Can you work these out from the model? Positions are in its coordinate system, mm. Give positions to 0.01 mm unless a question says otherwise; leave off trailing zeros. Write each loop counter-clockwise with the first axis right and the second up, starting at its lowest first coordinate (ties: lowest second). Pieces come first, ordered by that corner, then holes. Notation, with made-up numbers: M 50.5,-17.5 L 76.5,-17.5 A23 cw 76.5,7.5 Z; hole C -25,10 d5. An arc over 180 degrees is marked long. Write each question's results on one line, items separated by ' | '.
from build123d import *

# Parameters (mm, degrees)
SKETCH1_R           = 1.75
BOSS_EXTRUDE1_DEPTH = 4
SKETCH2_W           = 130
SKETCH2_H           = 10
BOSS_EXTRUDE2_DEPTH = 0.5
CUT_EXTRUDE1_DEPTH  = 2
SKETCH4_R           = 1.624205192
BOSS_EXTRUDE3_DEPTH = 4


with BuildPart() as part:
    # Sketch1 → Boss-Extrude1 (new body)
    with BuildSketch(Plane(origin=(0, 0, 0), x_dir=(1, 0, 0), z_dir=(0, 1, 0))):
        with BuildLine():
            ThreePointArc((75, 2), (74.121320344, 4.121320344), (72, 5))
            Line((72, 5), (-72, 5))
            ThreePointArc((-72, 5), (-74.121320344, 4.121320344), (-75, 2))
            Line((-75, 2), (-75, -5))
            Line((-75, -5), (75, -5))
            Line((75, -5), (75, 2))
        make_face()
        with Locations(Location((-70, 0, 0), (0, 0, 270))):
            Circle(SKETCH1_R, mode=Mode.SUBTRACT)
        with BuildLine():
            ThreePointArc((61.75, 0), (61.237436867, -1.237436867), (60, -1.75))
            Line((60, -1.75), (-60, -1.75))
            ThreePointArc((-60, -1.75), (-61.75, 0), (-60, 1.75))
            Line((-60, 1.75), (60, 1.75))
            ThreePointArc((60, 1.75), (61.237436867, 1.237436867), (61.75, 0))
        make_face(mode=Mode.SUBTRACT)
        with Locations(Location((70, 0, 0), (0, 0, 270))):
            Circle(SKETCH1_R, mode=Mode.SUBTRACT)
    extrude(amount=BOSS_EXTRUDE1_DEPTH)

    # Sketch2 → Boss-Extrude2 (add)
    with BuildSketch(Plane(origin=(0, 4, 0), x_dir=(1, 0, 0), z_dir=(0, 1, 0))):
        Rectangle(SKETCH2_W, SKETCH2_H)
        with BuildLine():
            Line((-60, 1.75), (60, 1.75))
            ThreePointArc((60, 1.75), (61.75, 0), (60, -1.75))
            Line((60, -1.75), (-60, -1.75))
            ThreePointArc((-60, -1.75), (-61.75, 0), (-60, 1.75))
        make_face(mode=Mode.SUBTRACT)
    extrude(amount=BOSS_EXTRUDE2_DEPTH)

    # Sketch3 → Cut-Extrude1 (cut)
    with BuildSketch(Plane.XY.offset(5)):
        with BuildLine():
            Line((58.5, 2.5), (-58.5, 2.5))
            ThreePointArc((-58.5, 2.5), (-59.560660172, 2.939339828), (-60, 4))
            Line((-60, 4), (-60, 4.5))
            Line((-60, 4.5), (60, 4.5))
            Line((60, 4.5), (60, 4))
            ThreePointArc((60, 4), (59.560660172, 2.939339828), (58.5, 2.5))
        make_face()
    extrude(amount=-CUT_EXTRUDE1_DEPTH, mode=Mode.SUBTRACT)

    # Sketch4 → Boss-Extrude3 (add)
    # profile 1 of 2: a face of its own
    with BuildSketch(Plane.XY.offset(5)):
        with BuildLine():
            Line((-75, 4), (-77, 6))
            ThreePointArc((-77, 6), (-82, 11), (-87, 6))
            Line((-87, 6), (-87, 0))
            Line((-87, 0), (-75, 0))
            Line((-75, 0), (-75, 4))
        make_face()
        with Locations((-82, 6)):
            Circle(SKETCH4_R, mode=Mode.SUBTRACT)
    # profile 2 of 2: a face of its own
    with BuildSketch(Plane.XY.offset(5)):
        with BuildLine():
            ThreePointArc((77, 6), (82, 11), (87, 6))
            Line((87, 6), (87, 0))
            Line((87, 0), (75, 0))
            Line((75, 0), (75, 4))
            Line((75, 4), (77, 6))
        make_face()
        with Locations((82, 6)):
            Circle(SKETCH4_R, mode=Mode.SUBTRACT)
    extrude(amount=-BOSS_EXTRUDE3_DEPTH)


solid = part.part
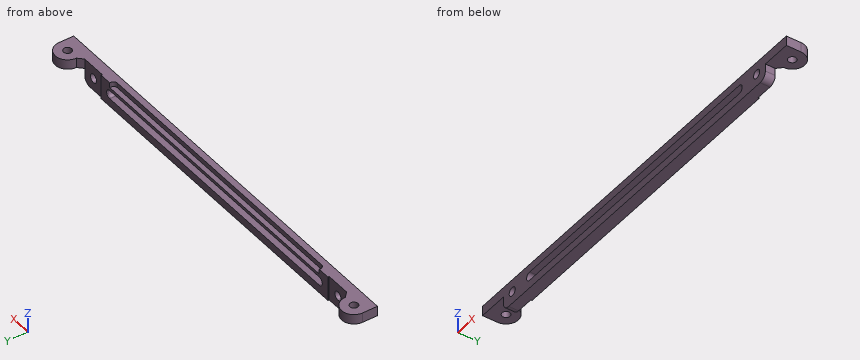
Item 1: I want a section at C-C, the plane y = 9.5. Please give me the cut outline in (x, z), and give its area (3 significant figures).
Geometry says:
outline: M -85.57,1 L -78.43,1 L -78.43,5 L -85.57,5 Z; M 78.43,1 L 85.57,1 L 85.57,5 L 78.43,5 Z | area: 57.1 mm2
Item 2: I want a section at A-A, the plane x = 82. Please give me the cut outline in (y, z).
Geometry says:
outline: M 0,1 L 4.38,1 L 4.38,5 L 0,5 Z; M 7.62,1 L 11,1 L 11,5 L 7.62,5 Z
Item 3: I want a section at B-B, the plane x = -37. Please give me the cut outline in (y, z).
Geometry says:
outline: M 0,-5 L 4.5,-5 L 4.5,-1.75 L 0,-1.75 Z; M 0,1.75 L 4.5,1.75 L 4.5,3 L 2.5,3 L 2.5,5 L 0,5 Z
Item 4: I'm going to push flat-ended pins straight in: pin 1 (6 mm diameter, centred on x = -44.5, y = 8.5, fed in from +Z); pin 2 (5.5 mm diameter, centred on x = -82, y = 7, fed in from -Z); pin 3 (5 mm diameter, centred on x = 70, z = -0.5, fed in from +Y). Where does each tip first touch, or does it pass through?
Geometry says:
pin 1: passes through | pin 2: stops at z = 1 | pin 3: stops at y = 4
Item 5: If I drill on line 1 (Z direction, x = 31.5, y = 3.75); line 2 (Z direction, x = -70, y = 2.15); line 3 (X direction, y = 7, z = 2.5), over which ranges is the centre line in solid material (lowest first)? Write a range as from..to.
Geometry says:
line 1: z = -5..-1.75, 1.75..3 | line 2: z = -5..-1.75, 1.75..5 | line 3: x = -86.9..-83.28, -80.72..-77.1, 77.1..80.72, 83.28..86.9
Item 6: I want a section at D-D, the plane z = -3.5. Please give me the cut outline in (x, y).
Geometry says:
outline: M -74.6,0 L 74.6,0 L 74.6,4 L 65,4 L 65,4.5 L -65,4.5 L -65,4 L -74.6,4 Z
